Could you check a few things on this model? Use its own coordinates, in mm. A direction names the side the tool comes from. Give positions to 0.01 mm unless a question says otherwise; leave off trailing zeros. Loops run counter-clockwise (first coordinate to the right, second up) from the corner with the lowest first, then second, coordinate; pieces in that order, holes last. Notation, with made-up numbers: M 62.25,-23.5 L 96.25,-23.5 A15 ccw 96.25,5.5 Z; hole C 87,37.25 d4. An arc over 180 degrees is marked long. Answer in a Markdown table with one row per item. Add a question column.
1. I'm going to push flat-ended pins straight in: pin 1 Ø3 at (y, z) = (16.5, 2.5) entering from -X; pin 2 Ø1 at (x, y) = (-3, -31.5) entering from +Z; pin 3 Ø4 at (x, y) = (-3, 25) entering from -Z. Where does each tip first touch, or does it pass through?
2. Thinking about a two-plate mould opening in Y: for faces 1 (the flat face through (0, 74.5, 0)), 2 (the cylindrical face through (-1.141, 68.406, 3.625)), 3 (the cylindrical face through (-3.905, 0.952, -0.867)), which applies, released by +Y, released by -Y, zero draft, split by the parting line, or undercut?
3. If we section it at B-B on x = 1.75: List the corners of the cut face in (y, z) for me.
4. I need wall thicknesses on line 1 along X through (y, z) = (64, -1.25); line 2 along Z through (x, y) = (2.5, 50); line 3 along X through (y, z) = (6, 0.5). Which ranges of each line are inside material? Lowest first, please. Write a range as from..to.
5. Which directions (+Z, -Z, +X, -X, +Y, -Y) give clear straight access to the entire face, cutting with the end or side of a thin tool? Please do faces 4 (the cylindrical face through (-1.141, -68.406, 3.625)), 5 (the cylindrical face through (-3.905, 71.69, -0.867)).
6. If we section it at A-A on z = -1: List the corners of the cut face in (x, y) for me, then the cut area to 3 significant figures.
7. If we section it at C-C on y = 18: List the corners of the cut face in (x, z) for me, then the cut area to 3 significant figures.
```python
from build123d import *

# Parameters (mm, degrees)
SKETCH_1_R      = 4
EXTRUDE_1_DEPTH = 74.5
SKETCH_3_W      = 5
SKETCH_3_H      = 0.8


with BuildPart() as part:
    # 草图1 → 凸台-拉伸1 (new, symmetric)
    with BuildSketch(Plane(origin=(0, 0, 0), x_dir=(1, 0, 0), z_dir=(0, 1, 0))):
        with Locations(Location((0, 0, 0), (0, 0, 270))):
            Circle(SKETCH_1_R)
    extrude(amount=EXTRUDE_1_DEPTH, both=True)

    # 草图3 → 切除-旋转1 (revolve, cut)
    with BuildSketch(Plane(origin=(0, 0, 0), x_dir=(0, 0, -1), z_dir=(1, 0, 0)), mode=Mode.PRIVATE) as cut_revolve_1_sk:
        with Locations((6.3, 68.4)):
            Rectangle(SKETCH_3_W, SKETCH_3_H)
    cut_revolve_1 = revolve(cut_revolve_1_sk.sketch.rotate(Axis((0, 74.5, 0), (0, -1, 0)), 180), axis=Axis((0, 74.5, 0), (0, -1, 0)), mode=Mode.SUBTRACT)

    # 镜向1: 切除-旋转1 across plane
    add(cut_revolve_1.mirror(Plane.ZX), mode=Mode.SUBTRACT)


solid = part.part
```
Results:
| question | item | result |
|---|---|---|
| 1 | pin 1 | x = -3.87 |
| 1 | pin 2 | z = 3.12 |
| 1 | pin 3 | z = -3.87 |
| 2 | face 1 | released by +Y |
| 2 | face 2 | undercut |
| 2 | face 3 | zero draft |
| 3 | outline | M -74.5,-3.6 L -68.8,-3.6 L -68.8,-3.37 L -68,-3.37 L -68,-3.6 L 68,-3.6 L 68,-3.37 L 68.8,-3.37 L 68.8,-3.6 L 74.5,-3.6 L 74.5,3.6 L 68.8,3.6 L 68.8,3.37 L 68,3.37 L 68,3.6 L -68,3.6 L -68,3.37 L -68.8,3.37 L -68.8,3.6 L -74.5,3.6 Z |
| 4 | line 1 | -3.8..3.8 |
| 4 | line 2 | -3.12..3.12 |
| 4 | line 3 | -3.97..3.97 |
| 5 | face 4 | none |
| 5 | face 5 | +Y, -Y |
| 6 | outline | M -3.87,-74.5 L 3.87,-74.5 L 3.87,-68.8 L 3.67,-68.8 L 3.67,-68 L 3.87,-68 L 3.87,68 L 3.67,68 L 3.67,68.8 L 3.87,68.8 L 3.87,74.5 L -3.87,74.5 L -3.87,68.8 L -3.67,68.8 L -3.67,68 L -3.87,68 L -3.87,-68 L -3.67,-68 L -3.67,-68.8 L -3.87,-68.8 Z |
| 6 | area | 1,150 mm2 |
| 7 | outline | C 0,0 d8 |
| 7 | area | 50.3 mm2 |
